```python
from build123d import *

# Parameters (mm, degrees)
BOSS_EXTRUDE1_DEPTH      = 482.6
BOSS_EXTRUDE1_DEPTH_BACK = 482.6
SKETCH2_R                = 57.15
SKETCH2_R_2              = 5.08
SKETCH2_R_3              = 31.75
CUT_EXTRUDE1_DEPTH       = 965.2
FILLET1_R                = 0.79375
FILLET2_R                = 3.571875


with BuildPart() as part:
    # Sketch1 → Boss-Extrude1 (new, two sides: drawn at the far end of the back side and taken through both)
    with BuildSketch(Plane.XY.offset(-BOSS_EXTRUDE1_DEPTH_BACK)):
        Polygon((0, 0), (100.80625, 0), (100.80625, -29.845), (119.9515, -29.845), (119.9515, -33.02), (97.63125, -33.02), (97.63125, -3.175), (-97.63125, -3.175), (-97.63125, -33.02), (-119.9515, -33.02), (-119.9515, -29.845), (-100.80625, -29.845), (-100.80625, 0), align=None)
    extrude(amount=BOSS_EXTRUDE1_DEPTH + BOSS_EXTRUDE1_DEPTH_BACK)

    # Sketch2 → Cut-Extrude1 (cut)
    with BuildSketch(Plane(origin=(0, 0, 0), x_dir=(1, 0, 0), z_dir=(0, 1, 0))):
        with Locations(Location((0, 0, 0), (0, 0, 270))):
            Circle(SKETCH2_R)
        with Locations(Location((57.15, 57.15, 0), (0, 0, 270))):
            Circle(SKETCH2_R_2)
        with Locations(Location((57.15, -57.15, 0), (0, 0, 270))):
            Circle(SKETCH2_R_2)
        with Locations(Location((-57.15, -57.15, 0), (0, 0, 270))):
            Circle(SKETCH2_R_2)
        with Locations(Location((-57.15, 57.15, 0), (0, 0, 270))):
            Circle(SKETCH2_R_2)
        with Locations(Location((0, -266.7, 0), (0, 0, 270))):
            Circle(SKETCH2_R_3)
        with Locations(Location((77.47, -241.3, 0), (0, 0, 270))):
            Circle(SKETCH2_R_2)
        with Locations(Location((77.47, -292.1, 0), (0, 0, 270))):
            Circle(SKETCH2_R_2)
        with Locations(Location((-25.4, -344.17, 0), (0, 0, 270))):
            Circle(SKETCH2_R_2)
        with Locations(Location((25.4, -344.17, 0), (0, 0, 270))):
            Circle(SKETCH2_R_2)
        with Locations(Location((-77.47, -241.3, 0), (0, 0, 270))):
            Circle(SKETCH2_R_2)
        with Locations(Location((-77.47, -292.1, 0), (0, 0, 270))):
            Circle(SKETCH2_R_2)
        with Locations(Location((25.4, -189.23, 0), (0, 0, 270))):
            Circle(SKETCH2_R_2)
        with Locations(Location((-25.4, -189.23, 0), (0, 0, 270))):
            Circle(SKETCH2_R_2)
        with Locations(Location((-25.4, 189.23, 0), (0, 0, 270))):
            Circle(SKETCH2_R_2)
        with Locations(Location((77.47, 241.3, 0), (0, 0, 270))):
            Circle(SKETCH2_R_2)
        with Locations(Location((25.4, 189.23, 0), (0, 0, 270))):
            Circle(SKETCH2_R_2)
        with Locations(Location((-77.47, 241.3, 0), (0, 0, 270))):
            Circle(SKETCH2_R_2)
        with Locations(Location((0, 266.7, 0), (0, 0, 270))):
            Circle(SKETCH2_R_3)
        with Locations(Location((77.47, 292.1, 0), (0, 0, 270))):
            Circle(SKETCH2_R_2)
        with Locations(Location((-77.47, 292.1, 0), (0, 0, 270))):
            Circle(SKETCH2_R_2)
        with Locations(Location((-25.4, 344.17, 0), (0, 0, 270))):
            Circle(SKETCH2_R_2)
        with Locations(Location((25.4, 344.17, 0), (0, 0, 270))):
            Circle(SKETCH2_R_2)
        with BuildLine():
            Line((-5.08, -458.47), (-5.08, -439.674))
            ThreePointArc((-5.08, -439.674), (0, -434.594), (5.08, -439.674))
            Line((5.08, -439.674), (5.08, -458.47))
            ThreePointArc((5.08, -458.47), (0, -463.55), (-5.08, -458.47))
        make_face()
        with BuildLine():
            Line((-5.08, 458.47), (-5.08, 439.674))
            ThreePointArc((-5.08, 439.674), (0, 434.594), (5.08, 439.674))
            Line((5.08, 439.674), (5.08, 458.47))
            ThreePointArc((5.08, 458.47), (0, 463.55), (-5.08, 458.47))
        make_face()
    extrude(amount=-CUT_EXTRUDE1_DEPTH, mode=Mode.SUBTRACT)

    # Fillet1
    fillet1_edges = [part.edges().sort_by_distance(p)[0] for p in [
        (100.80625, -29.845, 0),
        (97.63125, -3.175, 0),
        (-97.63125, -3.175, 0),
        (-100.80625, -29.845, 0),
    ]]
    fillet(fillet1_edges, radius=FILLET1_R)

    # Fillet2
    fillet2_edges = [part.edges().sort_by_distance(p)[0] for p in [
        (100.80625, 0, 0),
        (97.63125, -33.02, 0),
        (-97.63125, -33.02, 0),
        (-100.80625, 0, 0),
    ]]
    fillet(fillet2_edges, radius=FILLET2_R)


solid = part.part
```
Model file for the job. Use its own axes, mm. A direction names the side the tool comes from. Coordinates: 2 decimals unless noted, no trailing zeros. Order: outer loops, then holes, each group sorted by start corner. A loop starts at its lowest first (then second) coordinate and runs counter-clockwise, first axis right, second up. Notation, with made-up numbers: (-3.75, -40) - (7.25, -40) arc R30 ccw to (7.25, -17) - close; hole circle Ø1 at (78.25, 35). An arc over 180 degrees is marked (long way). Return JSON: item names as keys, results as strings. Group by question number.
1) Saw through at C-C, the plane z = 205.5. Write the cut outline in (x, y) (1 decimal).
2) Saw through at B-B, the plane y = -10. Write the cut outline in (x, z), plus the area to 3 significant figures.
3) Tool access for faces 1 (the flat face through (-97.631, -17, -7)), 2 (the flat face through (-100.806, -16, -7)), 3 (the flat face through (111, -29.845, -7)): list every direction of +Z, -Z, +X, -X, +Y, -Y with a clear straight run to the whole face (end or side of a thin tool).
4) Mould opens along X. For faces 4 (the flat face through (100.806, -16, -7)), 5 (the flat face through (66, -3.175, -7)), 6 (the flat face through (111, -33.02, -7)), 7 (the cylindrical face through (-19.319, -1.565, -291.896)) say: released by +X, released by -X, zero draft, split by the parting line, or undercut.
5) Probe line 1 (Z direction, x = -77, y = -2); line 2 (X direction, y = -26, z = -270.5); line 3 (X direction, y = -1.15, z = -292.1). List the from-to ranges inside material, lowest first. Write a range as from..to.
6) Flat gauge pins, fed straight in: P1, Ø4, axis at y = -21.5, z = -255, coming from the +X side; P2, Ø1.5, axis at x = 94.5, z = -291.5, coming from the -Y side (3 decimals); P3, Ø5.5, axis at x = 111.5, z = -6.5, coming from the +Y side (3 decimals); P4, Ø6, axis at x = -25.4, z = -189.23, coming from the +Y side. Where does each tip first touch, or does it go through?
Values found:
{
 "1": {"outline": "(-120, -33) - (-101.2, -33) arc R3.6 ccw to (-97.6, -29.4) - (-97.6, -4) arc R0.8 cw to (-96.8, -3.2) - (96.8, -3.2) arc R0.8 cw to (97.6, -4) - (97.6, -29.4) arc R3.6 ccw to (101.2, -33) - (120, -33) - (120, -29.8) - (101.6, -29.8) arc R0.8 cw to (100.8, -29.1) - (100.8, -3.6) arc R3.6 ccw to (97.2, 0) - (-97.2, 0) arc R3.6 ccw to (-100.8, -3.6) - (-100.8, -29.1) arc R0.8 cw to (-101.6, -29.8) - (-120, -29.8) - close"},
 "2": {"outline": "(-100.81, -482.6) - (-97.63, -482.6) - (-97.63, 482.6) - (-100.81, 482.6) - close; (97.63, -482.6) - (100.81, -482.6) - (100.81, 482.6) - (97.63, 482.6) - close", "area": "6,130 mm²"},
 "3": {"face 1": "+Z, -Z, -Y", "face 2": "+Z, -Z, -X, +Y", "face 3": "+Z, -Z, +X, +Y"},
 "4": {"face 4": "released by +X", "face 5": "undercut", "face 6": "zero draft", "face 7": "undercut"},
 "5": {"line 1": "z = -482.6..-297.16, -287.04..-246.36, -236.24..236.24, 246.36..287.04, 297.16..482.6", "line 2": "x = -100.81..-97.63, 97.63..100.81", "line 3": "x = -99.86..-82.55, -72.39..-19.05, 19.05..72.39, 82.55..99.86"},
 "6": {"P1": "stops at x = 100.81", "P2": "stops at y = -3.175", "P3": "stops at y = -29.845", "P4": "passes through"}
}
